Check sheet for the modelled part. Datum: model origin and axes. Units: mm. A direction names the side the tool comes from. Give positions to 0.01 mm unless a question says otherwise; leave off trailing zeros. Order: outer loops, then holes, each group sorted by start corner. A loop starts at its lowest first (then second) coordinate and runs counter-clockwise, first axis right, second up.
Item 1: Gauge pin test, flat ends, axial feed: P1, Ø10, axis at y = 24, z = 17, coming from the +X side; P2, Ø2, axis at x = 38, z = 111, coming from the +Y side; P3, Ø1.8, axis at y = -1.5, z = 112, coming from the -X side. Record the tip position at first contact, or that the pin passes through.
Item 2: Access from +Z, -Z, +X, -X, +Y, -Y to the whole of each face (thin tool, end or side, straight path). Record for faces 4 (the flat face through (3, 28.687, 54)), 5 (the cylindrical face through (-57.699, 33.014, 28.035)), 6 (the flat face through (3, 2.172, 111)).
Item 3: Material ranges on line 1 along Y through (x, z) = (-62.5, 58); line 2 along Y through (x, z) = (-68, 88); line 3 along Y through (x, z) = (-25.5, 20), recorded low to high.
Item 4: Release check for a two-part mould opening along Z. For faces 1 (the flat face through (39, 2.172, 111)), 2 (the flat face through (-33, -1, 114.8)), 3 (the cylindrical face through (-57.7, 33.01, 13.37)) record: released by +Z, released by -Z, zero draft, split by the parting line, or undercut.
Item 5: Sectioned sample at C-C on x = -51. Record the boundary of the cut face in (y, z).
Item 6: Sectioned sample at D-D on x = -28.5. Record the boundary of the cut face in (y, z), and give its area (3 significant figures).
Item 7: Sectioned sample at B-B on y = -12. Record the boundary of the cut face in (x, z), and give its area (3 significant figures).
Item 8: Sectioned sample at A-A on z = 94.5. Record the boundary of the cut face in (x, y).
from build123d import *

# Parameters (mm, degrees)
SKETCH_1_W               = 165
SKETCH_1_H               = 68
EXTRUDE_1_DEPTH          = 105.8
SKETCH_2_W               = 39.381596793
SKETCH_2_H               = 19.528929346
SKETCH_2_W_2             = 20.130205532
CUT_EXTRUDE_1_DEPTH      = 2
SKETCH_3_R               = 4.669286721
CUT_EXTRUDE_2_DEPTH      = 2
SKETCH_4_W               = 21.280991735
SKETCH_4_H               = 10.640495868
SKETCH_4_W_2             = 19.950929752
EXTRUDE_2_DEPTH          = 2
SKETCH_5_W               = 13.799393078
SKETCH_5_H               = 5.887741047
SKETCH_5_W_2             = 12.327457817
SKETCH_5_W_3             = 15.087336432
EXTRUDE_3_DEPTH          = 7
SKETCH_6_W               = 105.8
SKETCH_6_H               = 3.312578262
CUT_EXTRUDE_3_DEPTH      = 161
CUT_EXTRUDE_4_DEPTH      = 58
CUT_EXTRUDE_4_DEPTH_BACK = 58
SKETCH_7_W               = 16.710317156
SKETCH_7_H               = 19.528929346
SKETCH_8_W               = 20.11053719
SKETCH_8_H               = 105.021694215
CUT_EXTRUDE_5_DEPTH      = 58


with BuildPart() as part:
    # 草图1 → 凸台-拉伸1 (new body)
    with BuildSketch(Plane.XY):
        Rectangle(SKETCH_1_W, SKETCH_1_H)
    extrude(amount=EXTRUDE_1_DEPTH)

    # 草图2 → 切除-拉伸1 (cut)
    with BuildSketch(Plane(origin=(0, 34, 0), x_dir=(1, 0, 0), z_dir=(0, 1, 0))):
        with Locations((-62.809201604, -96.035535327)):
            Rectangle(SKETCH_2_W, SKETCH_2_H)
        with Locations((-33.053300441, -96.035535327)):
            Rectangle(SKETCH_2_W_2, SKETCH_2_H)
        Polygon((82.5, 0), (-43.118403207, 0), (-43.118403207, -86.271070654), (-22.988197675, -86.271070654), (-22.988197675, -105.8), (82.5, -105.8), align=None)
    extrude(amount=-CUT_EXTRUDE_1_DEPTH, mode=Mode.SUBTRACT)

    # 草图3 → 切除-拉伸2 (cut)
    with BuildSketch(Plane(origin=(0, 34, 0), x_dir=(1, 0, 0), z_dir=(0, 1, 0))):
        with Locations(Location((-53.556287556, -11.217711758, 0), (0, 0, 270))):
            Circle(SKETCH_3_R)
        with Locations(Location((-53.556287556, -25.880454059, 0), (0, 0, 270))):
            Circle(SKETCH_3_R)
        with Locations(Location((-53.556287556, -42.282843752, 0), (0, 0, 270))):
            Circle(SKETCH_3_R)
        with Locations(Location((-53.556287556, -55.205938661, 0), (0, 0, 270))):
            Circle(SKETCH_3_R)
        with Locations(Location((-53.556287556, -70.61424413, 0), (0, 0, 270))):
            Circle(SKETCH_3_R)
    extrude(amount=-CUT_EXTRUDE_2_DEPTH, mode=Mode.SUBTRACT)

    # 草图4 → 凸台-拉伸2 (add)
    with BuildSketch(Plane.XY.offset(105.8)):
        with Locations((-33.584065083, -0.665030992)):
            Rectangle(SKETCH_4_W, SKETCH_4_H)
        with Locations((1.662577479, -0.665030992)):
            Rectangle(SKETCH_4_W_2, SKETCH_4_H)
        with Locations((38.68263602, -0.665030992)):
            Rectangle(SKETCH_4_W, SKETCH_4_H)
    extrude(amount=EXTRUDE_2_DEPTH)

    # 草图5 → 凸台-拉伸3 (add)
    with BuildSketch(Plane.XY.offset(107.8)):
        with Locations((-33.115606168, -0.77221182)):
            Rectangle(SKETCH_5_W, SKETCH_5_H)
        with Locations((2.946807743, -0.77221182)):
            Rectangle(SKETCH_5_W_2, SKETCH_5_H)
        with Locations((38.733233794, -0.77221182)):
            Rectangle(SKETCH_5_W_3, SKETCH_5_H)
    extrude(amount=EXTRUDE_3_DEPTH)

    # 草图6 → 切除-拉伸3 (cut)
    with BuildSketch(Plane(origin=(82.5, 0, 0), x_dir=(0, 0, -1), z_dir=(1, 0, 0))):
        with Locations((-52.9, 30.343710869)):
            Rectangle(SKETCH_6_W, SKETCH_6_H)
    extrude(amount=-CUT_EXTRUDE_3_DEPTH, mode=Mode.SUBTRACT)

    # 草图7 → 切除-拉伸4 (cut, two sides: drawn at the far end of the back side and taken through both)
    with BuildSketch(Plane(origin=(0, 28.687421738, 0), x_dir=(1, 0, 0), z_dir=(0, 1, 0)).offset(-CUT_EXTRUDE_4_DEPTH_BACK)):
        with Locations((-74.144841422, -96.035535327)):
            Rectangle(SKETCH_7_W, SKETCH_7_H)
    extrude(amount=CUT_EXTRUDE_4_DEPTH + CUT_EXTRUDE_4_DEPTH_BACK, mode=Mode.SUBTRACT)

    # 草图8 → 切除-拉伸5 (cut)
    with BuildSketch(Plane(origin=(0, 28.687421738, 0), x_dir=(1, 0, 0), z_dir=(0, 1, 0))):
        with Locations((79.803719008, -58.198037191)):
            Rectangle(SKETCH_8_W, SKETCH_8_H)
    extrude(amount=-CUT_EXTRUDE_5_DEPTH, mode=Mode.SUBTRACT)


solid = part.part
Report:
1. P1: stops at x = 69.75
1. P2: stops at y = 2.17
1. P3: stops at x = -40.02
2. face 4: +Z, -Z, +X
2. face 5: +Y
2. face 6: +Z, +X, -X, +Y
3. line 1: y = -34 to 28.69, 32 to 34
3. line 2: y = -34 to -29.31
3. line 3: y = -34 to 28.69
4. face 1: zero draft
4. face 2: released by +Z
4. face 3: undercut
5. outline: (-34, 0) - (28.69, 0) - (28.69, 105.8) - (-34, 105.8) - close; (32, 0) - (34, 0) - (34, 7.31) - (32, 7.31) - close; (32, 15.13) - (34, 15.13) - (34, 21.97) - (32, 21.97) - close; (32, 29.79) - (34, 29.79) - (34, 38.38) - (32, 38.38) - close; (32, 46.19) - (34, 46.19) - (34, 51.3) - (32, 51.3) - close; (32, 59.11) - (34, 59.11) - (34, 66.71) - (32, 66.71) - close; (32, 74.52) - (34, 74.52) - (34, 86.27) - (32, 86.27) - close
6. outline: (-34, 0) - (28.69, 0) - (28.69, 105.8) - (4.66, 105.8) - (4.66, 107.8) - (2.17, 107.8) - (2.17, 114.8) - (-3.72, 114.8) - (-3.72, 107.8) - (-5.99, 107.8) - (-5.99, 105.8) - (-34, 105.8) - close
6. area: 6,690 mm2
7. outline: (-82.5, 0) - (82.5, 0) - (82.5, 5.69) - (69.75, 5.69) - (69.75, 105.8) - (-65.79, 105.8) - (-65.79, 86.27) - (-82.5, 86.27) - close
7. area: 15,900 mm2
8. outline: (-82.5, -34) - (82.5, -34) - (82.5, -29.31) - (69.75, -29.31) - (69.75, 28.69) - (-65.79, 28.69) - (-65.79, -29.31) - (-82.5, -29.31) - close
